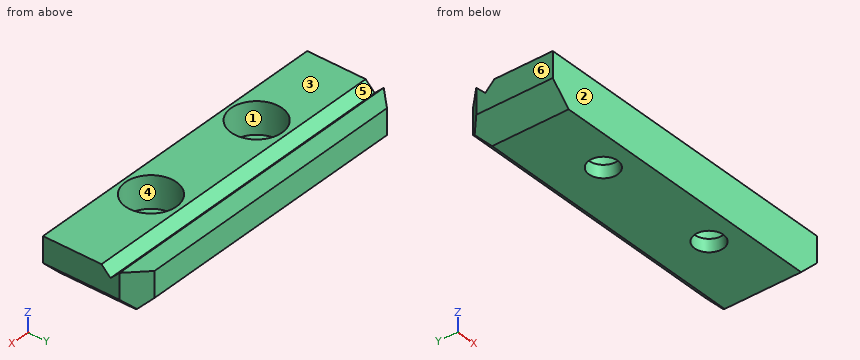
```python
from build123d import *

# Parameters (mm, degrees)
F1_DEPTH       = 7
F3_D           = 4.5
F3_CBORE_D     = 8
F3_CBORE_DEPTH = 5
F4_SIZE        = 3
F5_SIZE        = 3
F7_DEPTH       = 50


with BuildPart() as f1:
    # F0 (on Top) → F1 (new body)
    with BuildSketch(Plane.XY):
        Polygon((-20, -5), (20, -5), (25, -5), (25, 10), (20, 10), (-20, 10), (-25, 10), (-25, -5), align=None)
    extrude(amount=F1_DEPTH)

    # F3 (through all)
    with Locations(Plane.XY.offset(7)):
        with Locations((-10, -0.5), (10, -0.5)):
            CounterBoreHole(F3_D / 2, F3_CBORE_D / 2, F3_CBORE_DEPTH)

    # F4
    f4_edges = [f1.edges().sort_by_distance(p)[0] for p in [
        (-25, 10, 3.5),
        (25, 10, 3.5),
    ]]
    chamfer(f4_edges, length=F4_SIZE)

    # F5 (call 1 of 3: OpenCascade refuses the feature's edges together)
    f5_edges = [f1.edges().sort_by_distance(p)[0] for p in [
        (0, 10, 0),
    ]]
    chamfer(f5_edges, length=F5_SIZE)

    # F5#2 (call 2 of 3)
    f5_2_edges = [f1.edges().sort_by_distance(p)[0] for p in [
        (25, 1, 0),
    ]]
    chamfer(f5_2_edges, length=F5_SIZE)

    # F5#3 (call 3 of 3)
    f5_3_edges = [f1.edges().sort_by_distance(p)[0] for p in [
        (-25, 1, 0),
    ]]
    chamfer(f5_3_edges, length=F5_SIZE)

    # F6 (on face) → F7 (cut)
    with BuildSketch(Plane.YZ.offset(25)):
        Polygon((5.5857864376, 5.5857864376), (7, 7), (4.1715728753, 7), align=None)
    extrude(amount=-F7_DEPTH, mode=Mode.SUBTRACT)


solid = f1.part
```
Part model, mm, in its own coordinate system. Face numbers are marked on the shaded views. A direction names the side the tool comes from. Give positions to 0.01 mm unless a question says otherwise; leave off trailing zeros. Order: outer loops, then holes, each group sorted by start corner. A loop starts at its lowest first (then second) coordinate and runs counter-clockwise, first axis right, second up. Notation, with made-up numbers: (75.5, 44) - (105.5, 44) arc R14 ccw to (105.5, 63) - close; hole circle Ø7 at (88, 76). An arc over 180 degrees is marked (long way). Use one line per item in the form item = value.
Item 1: Probe probe 1 along Y at (x, z) = (10, 5.55); probe 2 along Y at (x, z) = (13.5, 6.5); probe 3 along Y at (x, z) = (22, 6.5). List the from-to ranges inside material, lowest first. Write a range as from..to.
Solution:
probe_1 = -5..-4.5, 3.5..10
probe_2 = -5..-2.44, 1.44..4.67, 6.5..10
probe_3 = -5..4.67, 6.5..10
Item 2: Which spindle directions (+Z, -Z, +X, -X, +Y, -Y) get a long thin tool onto all of the face, cutting with end or side? Do the marked faces 4, 5 and 6. Say none if no direction does.
Solution:
face_4 = +Z
face_5 = +Z, +X, -X
face_6 = +Z, -Z, -X, +Y, -Y
Item 3: Slice it at C-C on x = -10. Give the cut face in (y, z), and give its area (3 significant figures).
Solution:
outline = (-5, 0) - (-2.75, 0) - (-2.75, 2) - (-4.5, 2) - (-4.5, 7) - (-5, 7) - close; (1.75, 0) - (7, 0) - (10, 3) - (10, 7) - (7, 7) - (5.59, 5.59) - (4.17, 7) - (3.5, 7) - (3.5, 2) - (1.75, 2) - close
area = 49.5 mm2
Item 4: Pin check, flat tips, straight feed: pin 1 Ø4 at (x, z) = (-12.5, 2) entering from +Y; pin 2 Ø6 at (x, y) = (10, -0.5) entering from +Z. Stop position of each tip, or through.
Solution:
pin_1 = 10
pin_2 = 2
Item 5: Two-plate mould, pull along Y, no slides. Class the marked faces 1, 2 and 3: released by +Y, released by -Y, zero draft, split by the parting line, or undercut.
Solution:
face_1 = undercut
face_2 = released by -Y
face_3 = zero draft
Item 6: Slice it at D-D on x = -21.5. Give the cut face in (y, z).
Solution:
outline = (-5, 0) - (7, 0) - (10, 3) - (10, 7) - (7, 7) - (5.59, 5.59) - (4.17, 7) - (-5, 7) - close
Item 7: Slice it at A-A on z = 4.5. Give the cut face in (x, y).
Solution:
outline = (-25, -5) - (25, -5) - (25, 7) - (22, 10) - (-22, 10) - (-25, 7) - close; hole circle Ø8 at (-10, -0.5); hole circle Ø8 at (10, -0.5)
Item 8: Slice it at B-B on y = 0.25. Give the cut face in (x, z), and give its area (3 significant figures).
Solution:
outline = (-25, 3) - (-22, 0) - (-12.12, 0) - (-12.12, 2) - (-13.93, 2) - (-13.93, 7) - (-25, 7) - close; (-7.88, 0) - (7.88, 0) - (7.88, 2) - (6.07, 2) - (6.07, 7) - (-6.07, 7) - (-6.07, 2) - (-7.88, 2) - close; (12.12, 0) - (22, 0) - (25, 3) - (25, 7) - (13.93, 7) - (13.93, 2) - (12.12, 2) - close
area = 245 mm2
